from build123d import *

# Parameters (mm, degrees)
BOSS_EXTRUDE1_DEPTH = 30
CIRPATTERN1_COUNT   = 12
SKETCH4_R           = 1.5
CUT_EXTRUDE1_DEPTH  = 30
CIRPATTERN2_COUNT   = 12


with BuildPart() as part:
    # Sketch3 → Boss-Extrude1 (new body)
    with BuildSketch(Plane(origin=(0, 0, 0), x_dir=(0, 0, -1), z_dir=(1, 0, 0))):
        with BuildLine():
            Line((-14.25, 24.681724008), (-5.575, 9.656183252))
            ThreePointArc((-5.575, 9.656183252), (-4.611154785, 10.151834886), (-3.603740814, 10.551566336))
            Line((-3.603740814, 10.551566336), (-3.863098868, 11.519503771))
            Line((-3.863098868, 11.519503771), (-5.111933128, 11.854127903))
            Line((-5.111933128, 11.854127903), (-9.81401728, 19.998376555))
            ThreePointArc((-9.81401728, 19.998376555), (-9.96754629, 21.665151442), (-8.800363492, 22.864898915))
            ThreePointArc((-8.800363492, 22.864898915), (-6.341066605, 23.665182744), (-3.811111111, 24.201765062))
            ThreePointArc((-3.811111111, 24.201765062), (-2.200427421, 23.746344671), (-1.5, 22.226110771))
            Line((-1.5, 22.226110771), (-1.5, 12.821942467))
            Line((-1.5, 12.821942467), (-2.414210129, 11.907732339))
            Line((-2.414210129, 11.907732339), (-2.154852075, 10.939794904))
            ThreePointArc((-2.154852075, 10.939794904), (-1.082540259, 11.097324299), (0, 11.15))
            Line((0, 11.15), (0, 28.5))
            ThreePointArc((0, 28.5), (-7.376342785, 27.528886049), (-14.25, 24.681724008))
        make_face()
    boss_extrude1 = extrude(amount=BOSS_EXTRUDE1_DEPTH)

    # CirPattern1: Boss-Extrude1 ×12 about axis
    cirpattern1_axis = Axis((0, 0, 0), (1, 0, 0))
    for i in range(1, CIRPATTERN1_COUNT):
        add(boss_extrude1.rotate(cirpattern1_axis, i * 360 / CIRPATTERN1_COUNT))

    # Sketch4 → Cut-Extrude1 (cut)
    with BuildSketch(Plane(origin=(0, 0, 0), x_dir=(0, 0, -1), z_dir=(1, 0, 0))):
        with Locations((0, 28.5)):
            Circle(SKETCH4_R)
    cut_extrude1 = extrude(amount=CUT_EXTRUDE1_DEPTH, mode=Mode.SUBTRACT)

    # CirPattern2: Cut-Extrude1 ×12 about axis
    cirpattern2_axis = Axis((0, 0, 0), (1, 0, 0))
    for i in range(1, CIRPATTERN2_COUNT):
        add(cut_extrude1.rotate(cirpattern2_axis, i * 360 / CIRPATTERN2_COUNT), mode=Mode.SUBTRACT)


solid = part.part
The model under review builds one solid part; all positions refer to its coordinate system, in mm. A direction names the side the tool comes from. Round coordinates to 2 decimals unless told otherwise and drop trailing zeros. Loops run counter-clockwise (first coordinate to the right, second up) from the corner with the lowest first, then second, coordinate; pieces in that order, holes last. Notation, with made-up numbers: (-2.75, -7.75) -> (24.25, -7.75) arc R22 ccw to (24.25, 14.25) -> close; hole circle Ø4 at (36, 55). An arc over 180 degrees is marked (long way). Answer as CSV lines item,"result".
1) Tool access review of faces 1 (the face through (15, 0, -27)), 2 (the face through (14.79, -10.09, 14.48)): name each direction out of +Z, -Z, +X, -X, +Y, -Y from which nothing blocks a thin tool from reaching the whole face with its end or side.
Geometry results:
face 1,"-Z, +X, -X"
face 2,"+X, -X"
2) To check wall thickness, follow line 1 along Z through (x, y) = (14.25, -7.5); line 2 along Y through (x, z) = (28, 22); line 3 along Z through (x, y) = (12.5, -19). State the ranges of each line that lie inside material, in increasing order. Write a range as from..to.
Geometry results:
line 1,"z = -27.5..-23.32, -15.99..-8.56, 8.56..15.99, 23.32..27.5"
line 2,"y = -18.12..-9.81, -1.5..1.5, 9.81..18.12"
line 3,"z = -21.24..-15.47, -12.82..-9.24, -1.5..1.5, 9.24..12.82, 15.47..21.24"
3) Draft analysis for pull direction Y (two halves, no side actions). For faces 3 (the face through (14.79, 27.507, -7.457)), 4 (the face through (14.79, 10.03, 14.37)), state which applies: pulls with the +Y half, pulls with the -Y half, needs draft (parallel to the pull), parting line crosses it, or undercut.
Geometry results:
face 3,"pulls with the +Y half"
face 4,"undercut"
4) Add section A-A on y = -14.25. Write out the cut boundary in (x, z), plus the area to 3 significant figures.
Geometry results:
outline,"(0, -23.18) -> (30, -23.18) -> (30, -19.5) -> (0, -19.5) -> close; (0, -9.96) -> (30, -9.96) -> (30, -6.5) -> (0, -6.5) -> close; (0, -1.5) -> (30, -1.5) -> (30, 1.5) -> (0, 1.5) -> close; (0, 6.5) -> (30, 6.5) -> (30, 9.96) -> (0, 9.96) -> close; (0, 19.5) -> (30, 19.5) -> (30, 23.18) -> (0, 23.18) -> close"
area,"519 mm²"
5) For P1, Ø2, axis at x = 14, z = -6, coming from the +Y side; P2, Ø3, axis at x = 11.5, y = 17.5, coming from the -Z side; P3, Ø3, axis at x = 21, z = -15.5, coming from the +Y side; P4, Ø1, axis at y = -20, z = 14, coming from the -X side, all flat-tipped, find the tip position at first contact; note any pin that passes through.
Geometry results:
P1,"stops at y = 28.06"
P2,"stops at z = -23.58"
P3,"stops at y = 23.9"
P4,"stops at x = 0"
